Geometry: see drawing. Coordinates: mm, zero at the bounding-box minimum. Round coordinates to 2 decimals unless told otherwise and drop trailing zeros. Write each loop counter-clockwise with the first axis right and the second up, starting at its lowest first coordinate (ties: lowest second). Pieces come first, ordered by that corner, then holes.
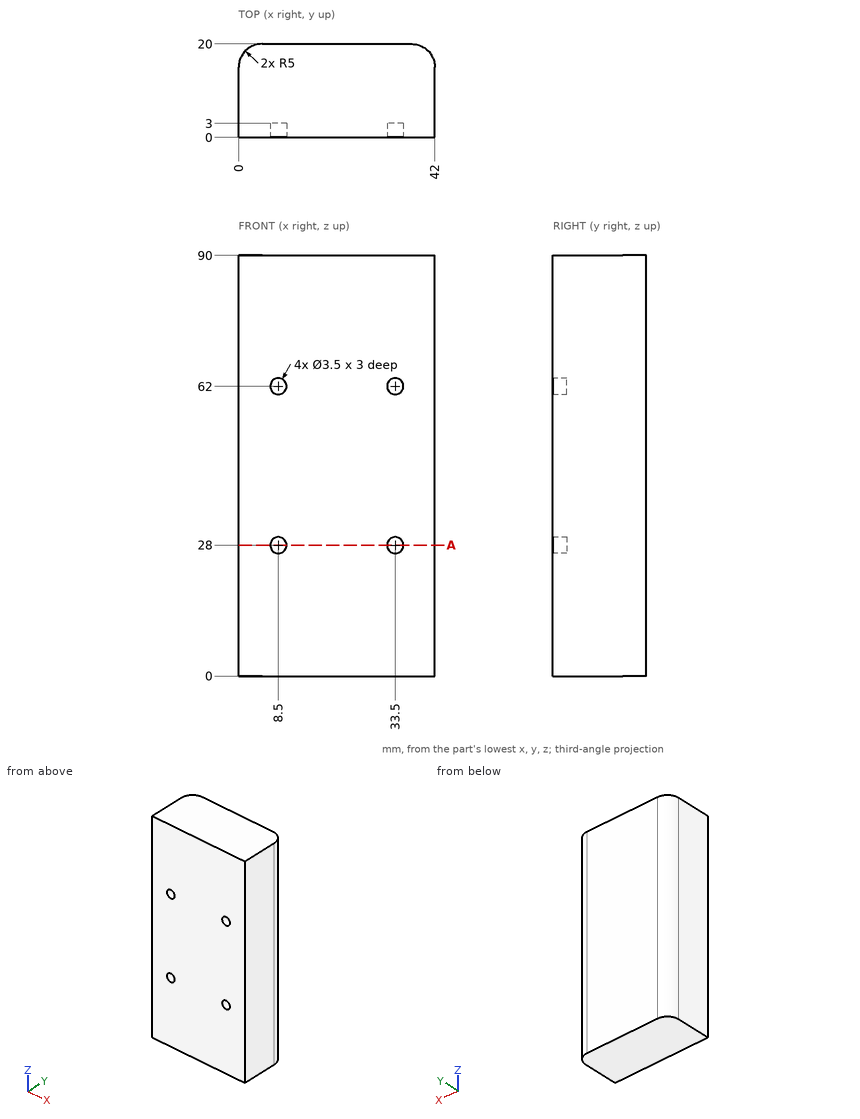
1) Contact query for flat-ended pins moving along their axis: P1, Ø1, axis at y = 17.5, z = 12, coming from the +X side; P2, Ø1, axis at x = 10, y = 3.5, coming from the -Z side; P3, Ø2, axis at x = 8.5, z = 28, coming from the -Y side. Output: stop coordinate, or through.
Taken from the geometry:
P1: stops at x = 41.58
P2: stops at z = 0
P3: stops at y = 3
2) Material intervals for line 1 (X direction, y = 1.85, z = 28); line 2 (X direction, y = 17, z = 31); line 3 (Y direction, x = 38, z = 37), sorted ascending.
Taken from the geometry:
line 1: x = 0 to 6.75, 10.25 to 31.75, 35.25 to 42
line 2: x = 0.42 to 41.58
line 3: y = 0 to 19.9
3) Section query A-A on z = 28. Return the cut outline in (x, y), then the cut area to 3 significant figures.
Taken from the geometry:
outline: (0, 0) - (6.75, 0) - (6.75, 3) - (10.25, 3) - (10.25, 0) - (31.75, 0) - (31.75, 3) - (35.25, 3) - (35.25, 0) - (42, 0) - (42, 15) arc R5 ccw to (37, 20) - (5, 20) arc R5 ccw to (0, 15) - close
area: 808 mm2
